Read the model definition and answer for the solid it produces. Units are mm, in the model's axes. A direction names the side the tool comes from. Coordinates: 2 decimals unless noted, no trailing zeros. Order: outer loops, then holes, each group sorted by start corner. A loop starts at its lowest first (then second) coordinate and runs counter-clockwise, first axis right, second up. Notation, with made-up numbers: (21, 34) - (68, 34) arc R19 ccw to (68, 70) - close; hole circle Ø1 at (23.25, -1). An arc over 180 degrees is marked (long way). Answer as a JSON object with one key per item and string values. Group by question number.
from build123d import *

# Parameters (mm, degrees)
CYLINDER018_R           = 5.9
CYLINDER018_DEPTH       = 13.8
CYLINDER020_R           = 0.6
CYLINDER020_DEPTH       = 16
CYLINDER021_R           = 0.6
CYLINDER021_DEPTH       = 16
BOX008_W                = 1.3
BOX008_H                = 2.6
BOX008_DEPTH            = 11
CYLINDER022_R           = 0.6
CYLINDER022_DEPTH       = 16
CYLINDER023_R           = 0.6
CYLINDER023_DEPTH       = 16
CYLINDER024_R           = 0.6
CYLINDER024_DEPTH       = 16
CYLINDER026_W           = 6.75
CYLINDER026_H           = 3
CYLINDER026_ANGLE       = 262
BOX010_W                = 4.4
BOX010_H                = 10.19
BOX010_DEPTH            = 2
CYLINDER027_R           = 6.75
CYLINDER027_DEPTH       = 1
BOX011_W                = 3
BOX011_H                = 0.55
BOX011_DEPTH            = 14
BOX012_W                = 3
BOX012_H                = 0.55
BOX012_DEPTH            = 14
BOX013_W                = 3
BOX013_H                = 0.55
BOX013_DEPTH            = 14
BOX014_W                = 3
BOX014_H                = 0.55
BOX014_DEPTH            = 14
BOX015_W                = 3
BOX015_H                = 0.55
BOX015_DEPTH            = 14
BOX007_W                = 5
BOX007_H                = 11
BOX007_DEPTH            = 3
BODY018_PLACEMENT_ANGLE = 90


with BuildPart() as part:
    # Cylinder018 → Cylinder018 (join)
    with BuildSketch(Plane.XY.offset(2)):
        Circle(CYLINDER018_R)
    extrude(amount=CYLINDER018_DEPTH)

    # Cylinder020 → Cylinder020 (cut)
    with BuildSketch(Plane(origin=(0, 3.5, 0), x_dir=(1, 0, 0), z_dir=(0, 0, 1))):
        Circle(CYLINDER020_R)
    extrude(amount=CYLINDER020_DEPTH, mode=Mode.SUBTRACT)

    # Cylinder021 → Cylinder021 (cut)
    with BuildSketch(Plane(origin=(0, -3.5, 0), x_dir=(1, 0, 0), z_dir=(0, 0, 1))):
        Circle(CYLINDER021_R)
    extrude(amount=CYLINDER021_DEPTH, mode=Mode.SUBTRACT)

    # Box008 → Box008 (cut)
    with BuildSketch(Plane(origin=(4.6, -1.3, 5), x_dir=(1, 0, 0), z_dir=(0, 0, 1))):
        with Locations((0.65, 1.3)):
            Rectangle(BOX008_W, BOX008_H)
    extrude(amount=BOX008_DEPTH, mode=Mode.SUBTRACT)

    # Cylinder022 → Cylinder022 (cut)
    with BuildSketch(Plane(origin=(-3, 0, 0), x_dir=(1, 0, 0), z_dir=(0, 0, 1))):
        Circle(CYLINDER022_R)
    extrude(amount=CYLINDER022_DEPTH, mode=Mode.SUBTRACT)

    # Cylinder023 → Cylinder023 (cut)
    with BuildSketch(Plane(origin=(-2.3, -2.3, 0), x_dir=(1, 0, 0), z_dir=(0, 0, 1))):
        Circle(CYLINDER023_R)
    extrude(amount=CYLINDER023_DEPTH, mode=Mode.SUBTRACT)

    # Cylinder024 → Cylinder024 (cut)
    with BuildSketch(Plane(origin=(-2.3, 2.3, 0), x_dir=(1, 0, 0), z_dir=(0, 0, 1))):
        Circle(CYLINDER024_R)
    extrude(amount=CYLINDER024_DEPTH, mode=Mode.SUBTRACT)

    # Cylinder026 → Cylinder026 (revolve)
    with BuildSketch(Plane(origin=(0, 0, 2), x_dir=(0.656059, 0.75471, 0), z_dir=(0.75471, -0.656059, 0))):
        with Locations((3.375, 1.5)):
            Rectangle(CYLINDER026_W, CYLINDER026_H)
    revolve(axis=Axis((0, 0, 2), (0, 0, 1)), revolution_arc=CYLINDER026_ANGLE)

    # Box010 → Box010 (join)
    with BuildSketch(Plane(origin=(0.03, -5.095, 2), x_dir=(1, 0, 0), z_dir=(0, 0, 1))):
        with Locations((2.2, 5.095)):
            Rectangle(BOX010_W, BOX010_H)
    extrude(amount=BOX010_DEPTH)

    # Cylinder027 → Cylinder027 (join)
    with BuildSketch(Plane.XY.offset(4.8)):
        Circle(CYLINDER027_R)
    extrude(amount=CYLINDER027_DEPTH)

    # Box011 → Box011 (cut)
    with BuildSketch(Plane(origin=(0.275, -5, 2), x_dir=(0, 1, 0), z_dir=(0, 0, 1))):
        with Locations((1.5, 0.275)):
            Rectangle(BOX011_W, BOX011_H)
    extrude(amount=BOX011_DEPTH, mode=Mode.SUBTRACT)

    # Box012 → Box012 (cut)
    with BuildSketch(Plane(origin=(-3.6, 3.2, 2), x_dir=(0.707107, -0.707107, 0), z_dir=(0, 0, 1))):
        with Locations((1.5, 0.275)):
            Rectangle(BOX012_W, BOX012_H)
    extrude(amount=BOX012_DEPTH, mode=Mode.SUBTRACT)

    # Box013 → Box013 (cut)
    with BuildSketch(Plane(origin=(-4.5, -0.25, 2), x_dir=(1, 0, 0), z_dir=(0, 0, 1))):
        with Locations((1.5, 0.275)):
            Rectangle(BOX013_W, BOX013_H)
    extrude(amount=BOX013_DEPTH, mode=Mode.SUBTRACT)

    # Box014 → Box014 (cut)
    with BuildSketch(Plane(origin=(-3.2, -3.6, 2), x_dir=(0.707107, 0.707107, 0), z_dir=(0, 0, 1))):
        with Locations((1.5, 0.275)):
            Rectangle(BOX014_W, BOX014_H)
    extrude(amount=BOX014_DEPTH, mode=Mode.SUBTRACT)

    # Box015 → Box015 (cut)
    with BuildSketch(Plane(origin=(0.275, 2, 2), x_dir=(0, 1, 0), z_dir=(0, 0, 1))):
        with Locations((1.5, 0.275)):
            Rectangle(BOX015_W, BOX015_H)
    extrude(amount=BOX015_DEPTH, mode=Mode.SUBTRACT)

    # Box007 → Box007 (cut)
    with BuildSketch(Plane(origin=(4.39, -5.5, 2), x_dir=(1, 0, 0), z_dir=(0, 0, 1))):
        with Locations((2.5, 5.5)):
            Rectangle(BOX007_W, BOX007_H)
    extrude(amount=BOX007_DEPTH, mode=Mode.SUBTRACT)


with BuildPart() as part_1:
    # Body018 placement: moved
    add(part.part.rotate(Axis((0, 0, 0), (0, 0, 1)), BODY018_PLACEMENT_ANGLE))


solid = part_1.part
1. A cutting plane is placed at B-B on y = 0. Write down the section's boundary in (x, z).
2. For a pull along Y with two mould halves and no side action, classify faces 1 (the flat face through (0, 0, 15.8)), 2 (the flat face through (0, 4.39, 3)), 3 (the flat face through (0.25, -2, 9)) as pulls with the +Y half, pulls with the -Y half, needs draft (parallel to the pull), parting line crosses it, or undercut.
3. For faces 4 (the flat face through (0, 4.6, 11)), 5 (the flat face through (3, -2.6, 8.8)), 6 (the cylindrical face through (-3.5, -0.6, 10.7)), determine the directions among +Z, -Z, +X, -X, +Y, -Y from which every point of the face is accessible in a straight line to the end or side of a thin tool.
4. A cutting plane is placed at D-D on z = 3. Write down the section's boundary in (x, y) (3 decimals), and give its area (3 significant figures).
5. A cutting plane is placed at A-A on x = 0. Write down the section's boundary in (y, z), and give its area (3 significant figures).
6. Straight lines are drawn through the part: L1, parallel to Y at x = 2.25, z = 13.5 (3 decimals); L2, parallel to X at y = -2, z = 9; L3, parallel to X at y = -1.25, z = 7.5. For each, find the intervals that lie inside material, in ascending order.
7. Given pin 1 (3.5 mm diameter, centred on x = 3.5, z = 12, fed in from -Y); pin 2 (6 mm diameter, centred on y = 3.5, z = 7, fed in from +X); pin 3 (8 mm diameter, centred on x = -4, z = 9, fed in from -Y), each flat-ended and moving along its own axis, determine where each tip first touches the part or whether it passes through.
8. A cutting plane is placed at C-C on y = -4. Write down the section's boundary in (x, z), and give its area (3 significant figures).
Derived:
{
 "1": {"outline": "(-6.75, 2) - (-5, 2) - (-5, 15.8) - (-5.9, 15.8) - (-5.9, 5.8) - (-6.75, 5.8) - close; (-2, 2) - (2, 2) - (2, 15.8) - (-2, 15.8) - close; (5, 2) - (6.75, 2) - (6.75, 5.8) - (5.9, 5.8) - (5.9, 15.8) - (5, 15.8) - close"},
 "2": {"face 1": "needs draft", "face 2": "pulls with the +Y half", "face 3": "undercut"},
 "3": {"face 4": "+Z, +Y", "face 5": "+Z, -Z", "face 6": "+Z"},
 "4": {"outline": "(-5.127, 4.39) arc R6.75 ccw (long way) to (5.127, 4.39) - close; hole (-5, -0.275) - (-2, -0.275) - (-2, 0.275) - (-5, 0.275) - close; hole (-3.589, -3.211) - (-3.2, -3.6) - (-1.079, -1.479) - (-1.468, -1.09) - close; hole (-0.3, -4.5) - (0.25, -4.5) - (0.25, -1.5) - (-0.3, -1.5) - close; hole (1.09, -1.468) - (3.211, -3.589) - (3.6, -3.2) - (1.479, -1.079) - close; hole (2, -0.275) - (5, -0.275) - (5, 0.275) - (2, 0.275) - close", "area": "118 mm2"},
 "5": {"outline": "(-6.75, 2) - (-4.5, 2) - (-4.5, 15.8) - (-5.9, 15.8) - (-5.9, 5.8) - (-6.75, 5.8) - close; (-1.5, 2) - (4.39, 2) - (4.39, 5) - (6.75, 5) - (6.75, 5.8) - (4.6, 5.8) - (4.6, 15.8) - (-1.5, 15.8) - close", "area": "108 mm2"},
 "6": {"L1": "y = -5.454 to -2.898, -1.702 to -0.275, 0.275 to 5.454", "L2": "x = -5.55 to -2.82, -1.6 to -0.3, 0.25 to 1.62, 2.82 to 5.55", "L3": "x = -5.77 to -1.63, -1.31 to 1.31, 1.65 to 5.77"},
 "7": {"pin 1": "stops at y = -5.63", "pin 2": "stops at x = 6.71", "pin 3": "stops at y = -6.56"},
 "8": {"outline": "(-5.44, 2) - (-0.3, 2) - (-0.3, 15.8) - (-4.34, 15.8) - (-4.34, 5.8) - (-5.44, 5.8) - close; (0.25, 2) - (5.44, 2) - (5.44, 5.8) - (4.34, 5.8) - (4.34, 15.8) - (0.25, 15.8) - close", "area": "120 mm2"}
}
